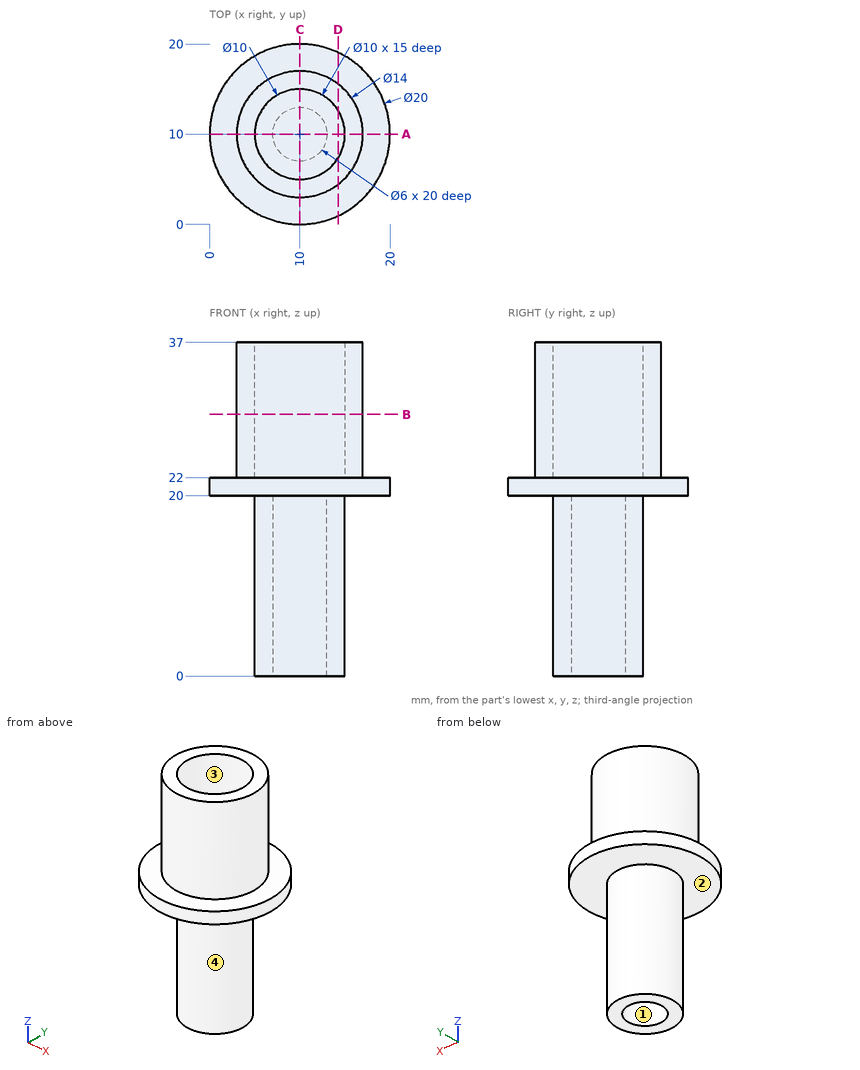
Check sheet for the drawn part. Datum: minimum x, y, z corner. Units: mm. Round coordinates to 2 decimals unless told otherwise and drop trailing zeros. Order: outer loops, then holes, each group sorted by start corner. A loop starts at its lowest first (then second) coordinate and runs counter-clockwise, first axis right, second up. Notation, with made-up numbers: M 56,-30 L 67,-30 A9 cw 67,-23 Z; hole C 85,-29 d8. An arc over 180 degrees is marked long. Answer in a Markdown table with one row per item.
(1) Section check A-A on y = 10. Record the boundary of the cut face in (x, z), plus the area to 3 significant figures.
Findings:
| item | result |
|---|---|
| outline | M 0,20 L 5,20 L 5,0 L 7,0 L 7,20 L 13,20 L 13,0 L 15,0 L 15,20 L 20,20 L 20,22 L 17,22 L 17,37 L 15,37 L 15,22 L 5,22 L 5,37 L 3,37 L 3,22 L 0,22 Z |
| area | 180 mm^2 |
(2) Draft check along Y on the marked faces 1, 2, 3 and 4. Enter one of: +Y half, -Y half, draft (parallel to the pull), parting line (faces both ways), or undercut.
Findings:
| item | result |
|---|---|
| face 1 | undercut |
| face 2 | draft |
| face 3 | undercut |
| face 4 | parting line |
(3) Gauge pin test, flat ends, axial feed: pin 1 (8 mm diameter, centred on x = 13.5, y = 17, fed in from -Z); pin 2 (3 mm diameter, centred on x = 16, z = 13.5, fed in from +Y); pin 3 (3 mm diameter, centred on x = 17.5, y = 16, fed in from -Z); pin 4 (1.5 mm diameter, centred on x = 7.5, y = 12.5, fed in from +Z). Record the tip position at first contact, or that the pin passes through.
Findings:
| item | result |
|---|---|
| pin 1 | stops at z = 0 |
| pin 2 | stops at y = 12.18 |
| pin 3 | stops at z = 20 |
| pin 4 | stops at z = 22 |
(4) Section check B-B on z = 29. Record the boundary of the cut face in (x, y).
Findings:
| item | result |
|---|---|
| outline | C 10,10 d14; hole C 10,10 d10 |
(5) Material ranges on line 1 along Y through (x, z) = (10, 13); line 2 along Y through (x, z) = (10, 25.5); line 3 along Z through (x, y) = (5.5, 2.75), recorded low to high. Write a range as from..to.
Findings:
| item | result |
|---|---|
| line 1 | y = 5..7, 13..15 |
| line 2 | y = 3..5, 15..17 |
| line 3 | z = 20..22 |
(6) Section check D-D on x = 14.25. Record the boundary of the cut face in (y, z), plus the area to 3 significant figures.
Findings:
| item | result |
|---|---|
| outline | M 0.95,20 L 7.37,20 L 7.37,0 L 12.63,0 L 12.63,20 L 19.05,20 L 19.05,22 L 15.56,22 L 15.56,37 L 12.63,37 L 12.63,22 L 7.37,22 L 7.37,37 L 4.44,37 L 4.44,22 L 0.95,22 Z |
| area | 229 mm^2 |
